The listing builds one solid part. Answer for the finished solid, in the listing's coordinates (mm). A direction names the side the tool comes from. Coordinates: 2 decimals unless noted, no trailing zeros. Order: outer loops, then holes, each group sorted by start corner. A loop starts at its lowest first (then second) coordinate and runs counter-clockwise, first axis right, second up. Notation, with made-up numbers: (19, -24.5) -> (61, -24.5) arc R19 ccw to (61, -4.5) -> close; hole circle Ø5 at (36.5, -36.75). An arc over 180 degrees is marked (long way). Write item = value, one per line.
from build123d import *

# Parameters (mm, degrees)
F0_W     = 92
F0_H     = 92
F0_R     = 2.15
F0_W_2   = 72
F0_H_2   = 72
F1_DEPTH = 1.5
F2_W     = 72
F2_H     = 3
F2_W_2   = 3
F2_H_2   = 72
F3_DEPTH = 1.5
F4_R     = 5
F5_R     = 0.75


with BuildPart() as f1:
    # F0 (on Front) → F1 (new body, symmetric)
    with BuildSketch(Plane.XZ):
        Rectangle(F0_W, F0_H)
        with Locations((-41, -41)):
            Circle(F0_R, mode=Mode.SUBTRACT)
        with Locations((41, -41)):
            Circle(F0_R, mode=Mode.SUBTRACT)
        with Locations((-41, 41)):
            Circle(F0_R, mode=Mode.SUBTRACT)
        Rectangle(F0_W_2, F0_H_2, mode=Mode.SUBTRACT)
        with Locations((41, 41)):
            Circle(F0_R, mode=Mode.SUBTRACT)
    extrude(amount=F1_DEPTH, both=True)

    # F2 (on face) → F3 (join)
    with BuildSketch(Plane(origin=(0, 1.5, 0), x_dir=(-1, 0, 0), z_dir=(0, 1, 0))):
        with Locations((0, 41)):
            Rectangle(F2_W, F2_H)
        with Locations((-41, 0)):
            Rectangle(F2_W_2, F2_H_2)
        with Locations((41, 0)):
            Rectangle(F2_W_2, F2_H_2)
        with Locations((0, -41)):
            Rectangle(F2_W, F2_H)
    extrude(amount=F3_DEPTH)

    # F4
    f4_edges = [f1.edges().sort_by_distance(p)[0] for p in [
        (-46, 0, 46),
        (46, 0, 46),
        (46, 0, -46),
        (-46, 0, -46),
        (36, 0, -36),
        (-36, 0, -36),
        (36, 0, 36),
        (-36, 0, 36),
    ]]
    fillet(f4_edges, radius=F4_R)

    # F5
    f5_edges = [f1.edges().sort_by_distance(p)[0] for p in [
        (39.5, 3, 0),
        (42.5, 3, 0),
        (41, 3, -36),
        (41, 3, 36),
        (0, 3, 42.5),
        (36, 3, 41),
        (0, 3, 39.5),
        (-36, 3, 41),
        (-41, 3, 36),
        (-39.5, 3, 0),
        (-42.5, 3, 0),
        (-41, 3, -36),
        (-36, 3, -41),
        (0, 3, -39.5),
        (36, 3, -41),
        (0, 3, -42.5),
    ]]
    fillet(f5_edges, radius=F5_R)


solid = f1.part
Q1. Each of these flat-tipped pins is pushed along its axis until it touches: pin 1 Ø7 at (x, z) = (-41, -41) entering from +Y; pin 2 Ø0.8 at (x, y) = (40.5, 2) entering from -Z; pin 3 Ø0.6 at (y, z) = (2, -14) entering from +X. Where does it stop, or does it pass through?
The answers:
pin_1 = 1.5
pin_2 = -36
pin_3 = 42.5
Q2. Section B-B, the plane y = -0.1 is taken. Give the vertices of the cut face in (x, z).
The answers:
outline = (-46, -41) arc R5 ccw to (-41, -46) -> (41, -46) arc R5 ccw to (46, -41) -> (46, 41) arc R5 ccw to (41, 46) -> (-41, 46) arc R5 ccw to (-46, 41) -> close; hole circle Ø4.3 at (-41, -41); hole circle Ø4.3 at (-41, 41); hole (-36, -31) arc R5 ccw to (-31, -36) -> (31, -36) arc R5 ccw to (36, -31) -> (36, 31) arc R5 ccw to (31, 36) -> (-31, 36) arc R5 ccw to (-36, 31) -> close; hole circle Ø4.3 at (41, -41); hole circle Ø4.3 at (41, 41)
Q3. Section A-A, the plane x = 24 is taken. Give the vertices of the cut face in (y, z).
The answers:
outline = (-1.5, -46) -> (1.5, -46) -> (1.5, -42.5) -> (2.25, -42.5) arc R0.75 ccw to (3, -41.75) -> (3, -40.25) arc R0.75 ccw to (2.25, -39.5) -> (1.5, -39.5) -> (1.5, -36) -> (-1.5, -36) -> close; (-1.5, 36) -> (1.5, 36) -> (1.5, 39.5) -> (2.25, 39.5) arc R0.75 ccw to (3, 40.25) -> (3, 41.75) arc R0.75 ccw to (2.25, 42.5) -> (1.5, 42.5) -> (1.5, 46) -> (-1.5, 46) -> close
Q4. Find the intervals of material crossed by line 1 along Z through (x, y) = (41, -0.05); line 2 along Z through (x, y) = (19, 2.4); line 3 along X through (y, z) = (1.2, -22), in increasing order.
The answers:
line_1 = -46 to -43.15, -38.85 to 38.85, 43.15 to 46
line_2 = -42.48 to -39.52, 39.52 to 42.48
line_3 = -46 to -36, 36 to 46
Q5. A tool of negligible diameter and unlimited length cuts with its end or side. For faces 1 (the face through (0, 0, 36)), 2 (the face through (-38, -1.5, 4)), from which of +Z, -Z, +X, -X, +Y, -Y can it reach the whole face along a straight path? Write none if from no direction.
The answers:
face_1 = +Y, -Y
face_2 = +Z, -Z, +X, -X, -Y
Q6. The mould has two halves that part along Z. Classify faces 3 (the face through (-46, 0, -1)), 4 (the face through (-1, 0, -46)), 5 (the face through (-45, 0, 44)), 6 (the face through (36, 0, 0)): released by +Z, released by -Z, zero draft, split by the parting line, or undercut.
The answers:
face_3 = zero draft
face_4 = released by -Z
face_5 = released by +Z
face_6 = undercut
Q7. Section C-C, the plane z = -25 is taken. Give the vertices of the cut face in (x, y), plus the area to 3 significant figures.
The answers:
outline = (-46, -1.5) -> (-36, -1.5) -> (-36, 1.5) -> (-39.5, 1.5) -> (-39.5, 2.25) arc R0.75 ccw to (-40.25, 3) -> (-41.75, 3) arc R0.75 ccw to (-42.5, 2.25) -> (-42.5, 1.5) -> (-46, 1.5) -> close; (36, -1.5) -> (46, -1.5) -> (46, 1.5) -> (42.5, 1.5) -> (42.5, 2.25) arc R0.75 ccw to (41.75, 3) -> (40.25, 3) arc R0.75 ccw to (39.5, 2.25) -> (39.5, 1.5) -> (36, 1.5) -> close
area = 68.5 mm2
